Geometry check sheet. Reference: the model listing, model coordinates, mm. A direction names the side the tool comes from. Round coordinates to 2 decimals unless told otherwise and drop trailing zeros. Order: outer loops, then holes, each group sorted by start corner. A loop starts at its lowest first (then second) coordinate and runs counter-clockwise, first axis right, second up.
(1) Set-up check for faces 4 (the face through (0, 2.65, -2)), 5 (the face through (-5.607, 0, -2)): record each of +Z, -Z, +X, -X, +Y, -Y from which the full face is reachable in a straight line by a thin tool's end or side.
(2) Cross-section at D-D on y = 1. Enter the section's corners in (x, z), and give its area (3 significant figures).
(3) Thickness scan on L1, parallel to Y at x = -1.25, z = -0.6; L2, parallel to X at y = 3.25, z = -2.7; L3, parallel to Y at x = -3, z = -1.95. Record the ranges inside material, lowest first.
(4) Cross-section at C-C on x = -0.25. Enter the section's corners in (y, z), and give its area (3 significant figures).
(5) Draft check along Y on faces 1 (the face through (-3, 1, 0)), 2 (the face through (3.115, 0.381, -1.972)), 3 (the face through (0, 5, -2)). Enter one of: pulls with the +Y half, pulls with the -Y half, needs draft (parallel to the pull), parting line crosses it, or undercut.
(6) Cross-section at A-A on z = -2.1. Enter the section's corners in (x, y).
(7) Cross-section at B-B on y = 3. Enter the section's corners in (x, z).
from build123d import *

# Parameters (mm, degrees)
F1_W     = 11.2149509114
F1_H     = 10
F2_DEPTH = 4
F4_DEPTH = 4


with BuildPart() as f2:
    # F1 (on Top) → F2 (new body)
    with BuildSketch(Plane.XY):
        Rectangle(F1_W, F1_H)
    extrude(amount=-F2_DEPTH)

    # F3 (on Top) → F4 (cut)
    with BuildSketch(Plane.XY):
        with BuildLine():
            ThreePointArc((2.5420287133, -2.4780213923), (3.2883660025, -1.3375907572), (3.55, 0))
            ThreePointArc((3.55, 0), (3.5407601901, 0.2559634273), (3.5130888585, 0.5105944302))
            Line((3.5130888585, 0.5105944302), (2.7057099648, 0.2482611253))
            Line((2.7057099648, 0.2482611253), (2.3348895716, 1.3895289449))
            Line((2.3348895716, 1.3895289449), (3.1422684653, 1.6518622498))
            ThreePointArc((3.1422684653, 1.6518622498), (2.0866376456, 2.87201033), (0.6, 3.4989284074))
            Line((0.6, 3.4989284074), (0.6, 2.65))
            Line((0.6, 2.65), (-0.6, 2.65))
            Line((-0.6, 2.65), (-0.6, 3.4989284074))
            ThreePointArc((-0.6, 3.4989284074), (-2.0866376456, 2.87201033), (-3.1422684653, 1.6518622498))
            Line((-3.1422684653, 1.6518622498), (-2.3348895716, 1.3895289449))
            Line((-2.3348895716, 1.3895289449), (-2.7057099648, 0.2482611253))
            Line((-2.7057099648, 0.2482611253), (-3.5130888585, 0.5105944302))
            ThreePointArc((-3.5130888585, 0.5105944302), (-3.3762506328, -1.09701033), (-2.5420287133, -2.4780213923))
            Line((-2.5420287133, -2.4780213923), (-2.0430411152, -1.7912238837))
            Line((-2.0430411152, -1.7912238837), (-1.072220722, -2.4965661865))
            Line((-1.072220722, -2.4965661865), (-1.5712083201, -3.1833636951))
            ThreePointArc((-1.5712083201, -3.1833636951), (0, -3.55), (1.5712083201, -3.1833636951))
            Line((1.5712083201, -3.1833636951), (1.072220722, -2.4965661865))
            Line((1.072220722, -2.4965661865), (2.0430411152, -1.7912238837))
            Line((2.0430411152, -1.7912238837), (2.5420287133, -2.4780213923))
        make_face()
    extrude(amount=-F4_DEPTH, mode=Mode.SUBTRACT)


solid = f2.part
Found:
1. face 4: +Z, -Z
1. face 5: +Z, -Z, -X, +Y, -Y
2. outline: (-5.61, -4) - (-2.46, -4) - (-2.46, 0) - (-5.61, 0) - close; (2.46, -4) - (5.61, -4) - (5.61, 0) - (2.46, 0) - close
2. area: 25.2 mm2
3. L1: y = -5 to -3.32, -2.74 to -2.37, 3.32 to 5
3. L2: x = -5.61 to -1.43, -0.6 to 0.6, 1.43 to 5.61
3. L3: y = -5 to -1.9, 0.34 to 1.61, 1.9 to 5
4. outline: (-5, -4) - (-3.54, -4) - (-3.54, 0) - (-5, 0) - close; (2.65, -4) - (5, -4) - (5, 0) - (2.65, 0) - close
4. area: 15.2 mm2
5. face 1: needs draft
5. face 2: undercut
5. face 3: pulls with the +Y half
6. outline: (-5.61, -5) - (5.61, -5) - (5.61, 5) - (-5.61, 5) - close; hole (-3.51, 0.51) arc R3.55 ccw to (-2.54, -2.48) - (-2.04, -1.79) - (-1.07, -2.5) - (-1.57, -3.18) arc R3.55 ccw to (1.57, -3.18) - (1.07, -2.5) - (2.04, -1.79) - (2.54, -2.48) arc R3.55 ccw to (3.51, 0.51) - (2.71, 0.25) - (2.33, 1.39) - (3.14, 1.65) arc R3.55 ccw to (0.6, 3.5) - (0.6, 2.65) - (-0.6, 2.65) - (-0.6, 3.5) arc R3.55 ccw to (-3.14, 1.65) - (-2.33, 1.39) - (-2.71, 0.25) - close
7. outline: (-5.61, -4) - (-1.9, -4) - (-1.9, 0) - (-5.61, 0) - close; (-0.6, -4) - (0.6, -4) - (0.6, 0) - (-0.6, 0) - close; (1.9, -4) - (5.61, -4) - (5.61, 0) - (1.9, 0) - close
